```python
from build123d import *

# Parameters (mm, degrees)
F0_W     = 30
F0_H     = 10
F1_DEPTH = 10
F2_R     = 3.7
F3_DEPTH = 10
F4_R     = 3.7
F5_DEPTH = 10
F6_R     = 2.99999


# Not quite as in the source:
# - a fillet or chamfer is up to 0.001 mm smaller than in the source, because OpenCascade refuses the exact size


with BuildPart() as f1:
    # F0 (on Top) → F1 (new body)
    with BuildSketch(Plane.XY):
        Rectangle(F0_W, F0_H)
    extrude(amount=F1_DEPTH)

    # F2 (on face) → F3 (cut, through all)
    with BuildSketch(Plane.XY.offset(10)):
        with Locations((8.3, 0)):
            Circle(F2_R)
    extrude(amount=-F3_DEPTH, mode=Mode.SUBTRACT)

    # F4 (on face) → F5 (cut, through all)
    with BuildSketch(Plane.XZ.offset(5)):
        with Locations((-8.7227521392, 5)):
            Circle(F4_R)
    extrude(amount=-F5_DEPTH, mode=Mode.SUBTRACT)

    # F6 (radius 3 in the source; OpenCascade refuses exactly that, so slightly less here)
    f6_edges = [f1.edges().sort_by_distance(p)[0] for p in [
        (-15, 0, 10),
        (15, 0, 10),
        (15, 0, 0),
        (-15, 0, 0),
    ]]
    fillet(f6_edges, radius=F6_R)


solid = f1.part
```
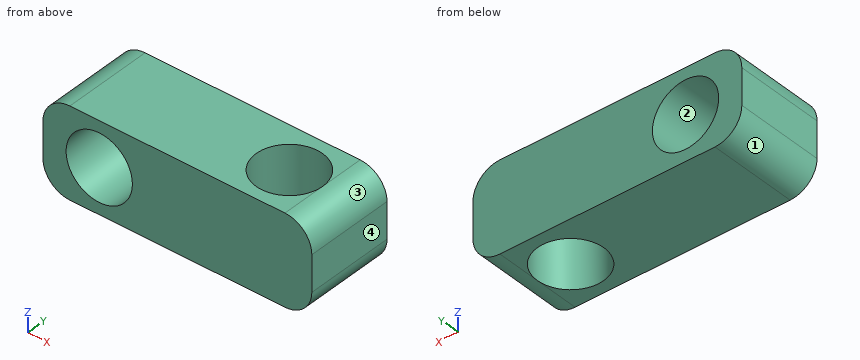
Geometry check sheet. Reference: the model listing, model coordinates, mm. Face numbers are marked on the shaded views. Give positions to 0.01 mm unless a question says otherwise; leave off trailing zeros. Order: outer loops, then holes, each group sorted by start corner. A loop starts at its lowest first (then second) coordinate and runs counter-clockwise, first axis right, second up.
1. Section check B-B, the plane y = 0. Give the number of separate pieces and of enclosed holes in the cut face, and give its area (3 significant figures).
2. Section check C-C, the plane x = 8.3. Enter the section's corners in (y, z).
3. Thickness scan on L1, parallel to Y at x = 8.3, z = 3.5; L2, parallel to X at y = 2.25, z = 3; L3, parallel to X at y = 0.5, z = 4.5. Record the ranges inside material, lowest first.
4. Section check D-D, the plane z = 8.25. Enter the section's corners in (x, y).
5. Gauge pin test, flat end, axial feed: pin 1 Ø6 at (x, z) = (-8.72, 5) entering from +Y. Record the tip position at first contact, or that the pin passes through.
6. Release check for a two-part mould opening along Z. For the marked faces 1, 2, 3 and 4 record: pulls with the +Z half, pulls with the -Z half, needs draft (parallel to the pull), parting line crosses it, or undercut.
7. Section check A-A, the plane z = 5. Enter the section's corners in (x, y), and give its area (3 significant figures).
Values follow:
1. separate pieces: 2
1. enclosed holes: 1
1. area: 175 mm2
2. outline: (-5, 0) - (-3.7, 0) - (-3.7, 10) - (-5, 10) - close; (3.7, 0) - (5, 0) - (5, 10) - (3.7, 10) - close
3. L1: y = -5 to -3.7, 3.7 to 5
3. L2: x = -15 to -11.84, -5.61 to 5.36, 11.24 to 15
3. L3: x = -15 to -12.39, -5.06 to 4.63, 11.97 to 15
4. outline: (-14.73, -5) - (-10.49, -5) - (-10.49, 5) - (-14.73, 5) - close; (-6.95, -5) - (14.73, -5) - (14.73, 5) - (-6.95, 5) - close; hole circle Ø7.4 at (8.3, 0)
5. pin 1: passes through
6. face 1: pulls with the -Z half
6. face 2: undercut
6. face 3: pulls with the +Z half
6. face 4: needs draft
7. outline: (-15, -5) - (-12.42, -5) - (-12.42, 5) - (-15, 5) - close; (-5.02, -5) - (15, -5) - (15, 5) - (-5.02, 5) - close; hole circle Ø7.4 at (8.3, 0)
7. area: 183 mm2
